Geometry: final body of the model. Coordinates: model frame, mm. Round coordinates to 2 decimals unless told otherwise and drop trailing zeros. Order: outer loops, then holes, each group sorted by start corner. A loop starts at its lowest first (then second) coordinate and runs counter-clockwise, first axis right, second up. Notation, with made-up numbers: M 37,35.25 L 58,35.25 A24 cw 58,67.25 Z; hole C 52,1.25 d6. An arc over 180 degrees is marked long. Return JSON: item names as keys, results as strings. Group by question number.
Q1. Cut plane A-A on z = -2.25. Output: boundary loops of the cut face in (x, y), and give its area (3 significant figures).
Q2. Mould query, pull axis Y, two halves, no side actions, for faces 1 (the face through (-18, 30.481, 0)), 2 (the face through (-21.58, -8.15, -0.13)), 3 (the face through (-19, -4, -10)). Classes: released by +Y, released by -Y, zero draft, split by the parting line, or undercut.
Q3. Cut plane B-B on x = -17. Count the separate pieces of the cut face and the enclosed holes in it, and give its area (3 significant figures).
Q4. Cut plane C-C on x = -0.5. Output: boundary loops of the cut face in (y, z), and give its area (3 significant figures).
Q5. Ray query, probe 1 along X at (y, z) = (-11, 1.25); probe 2 along Y at (x, z) = (-16, 5.5); probe 3 along X at (y, z) = (17, -3.5). Return the intervals inside material, ascending.
```python
from build123d import *

# Parameters (mm, degrees)
SKETCH1_R           = 10.25
SKETCH1_R_2         = 4.25
BOSS_EXTRUDE1_DEPTH = 10
CHAMFER1_SIZE       = 0.5
CHAMFER2_SIZE       = 0.5


with BuildPart() as part:
    # Sketch1 → Boss-Extrude1 (new, symmetric)
    with BuildSketch(Plane.XY):
        with BuildLine():
            Line((-7.444896481, 30.480652594), (-29.444896481, 30.480652594))
            ThreePointArc((-29.444896481, 30.480652594), (-36.515964293, 27.551720406), (-39.444896481, 20.480652594))
            Line((-39.444896481, 20.480652594), (-39.444896481, -26.519347406))
            Line((-39.444896481, -26.519347406), (2.555103519, -26.519347406))
            Line((2.555103519, -26.519347406), (2.555103519, 20.480652594))
            ThreePointArc((2.555103519, 20.480652594), (-0.373828669, 27.551720406), (-7.444896481, 30.480652594))
        make_face()
        with Locations((-18.444896481, 9.480652594)):
            Circle(SKETCH1_R, mode=Mode.SUBTRACT)
        with Locations((-18.444896481, -11.019347406)):
            Circle(SKETCH1_R_2, mode=Mode.SUBTRACT)
    extrude(amount=BOSS_EXTRUDE1_DEPTH, both=True)

    # Chamfer1
    chamfer1_edges = [part.edges().sort_by_distance(p)[0] for p in [
        (-28.694896481, 9.480652594, -10),
        (-28.694896481, 9.480652594, 10),
    ]]
    chamfer(chamfer1_edges, length=CHAMFER1_SIZE)

    # Chamfer2
    chamfer2_edges = [part.edges().sort_by_distance(p)[0] for p in [
        (-22.694896481, -11.019347406, -10),
        (-22.694896481, -11.019347406, 10),
    ]]
    chamfer(chamfer2_edges, length=CHAMFER2_SIZE)


solid = part.part
```
Result sheet:
{
 "1": {"outline": "M -39.44,-26.52 L 2.56,-26.52 L 2.56,20.48 A10 ccw -7.44,30.48 L -29.44,30.48 A10 ccw -39.44,20.48 Z; hole C -18.44,9.48 d20.5; hole C -18.44,-11.02 d8.5", "area": "1,960 mm²"},
 "2": {"face 1": "released by +Y", "face 2": "undercut", "face 3": "zero draft"},
 "3": {"separate pieces": "3", "enclosed holes": "0", "area": "573 mm²"},
 "4": {"outline": "M -26.52,-10 L 27.68,-10 L 27.68,10 L -26.52,10 Z", "area": "1,080 mm²"},
 "5": {"probe 1": "x = -39.44 to -22.69, -14.19 to 2.56", "probe 2": "y = -26.52 to -14.5, -7.54 to -0.47, 19.43 to 30.48", "probe 3": "x = -39.44 to -25.41, -11.48 to 2.56"}
}
